Answer from the drawing. Dimensions are ordinates in mm from the lowest x, y and z of the part. A direction names the side the tool comes from. Coordinates: 2 decimals unless noted, no trailing zeros. Write each loop counter-clockwise with the first axis right and the second up, starting at its lowest first coordinate (ties: lowest second). Pieces come first, ordered by that corner, then holes.
1) The part is cut by section B-B (y = 10). Determine the outline of the cut face in (x, z).
2) Find the intervals of material crossed by line 1 (X direction, y = 9.25, z = 13); line 2 (Y direction, x = 12.7, z = 11.5); line 3 (Y direction, x = 15.5, z = 9.5), in increasing order.
3) Which of the six approach directions +Z, -Z, +X, -X, +Y, -Y give full straight-line access (tool end or side, diameter ignored) to the marked faces 1, 2 and 3?
4) The part is cut by section C-C (x = 21.5). Determine the outline of the cut face in (y, z).
5) Each of these flat-tipped pins is pushed along its axis until it touches: pin 1 Ø6 at (x, z) = (10, 5.5) entering from +Y; pin 2 Ø1.9 at (y, z) = (6, 7.5) entering from +X; pin 3 Ø3 at (y, z) = (6, 5) entering from -X; pin 4 Ø5.5 at (x, z) = (3.048, 7.62) entering from +Y. Where does it stop, or does it pass through?
6) The part is cut by section A-A (z = 9.5). Give the number of separate pieces and of enclosed holes in the cut face, then the cut area to 3 significant figures.
7) Determine the mould class of the marked faces 4, 5 and 6 for opening direction X: +X half, -X half, draft (parallel to the pull), parting line (faces both ways), or undercut.
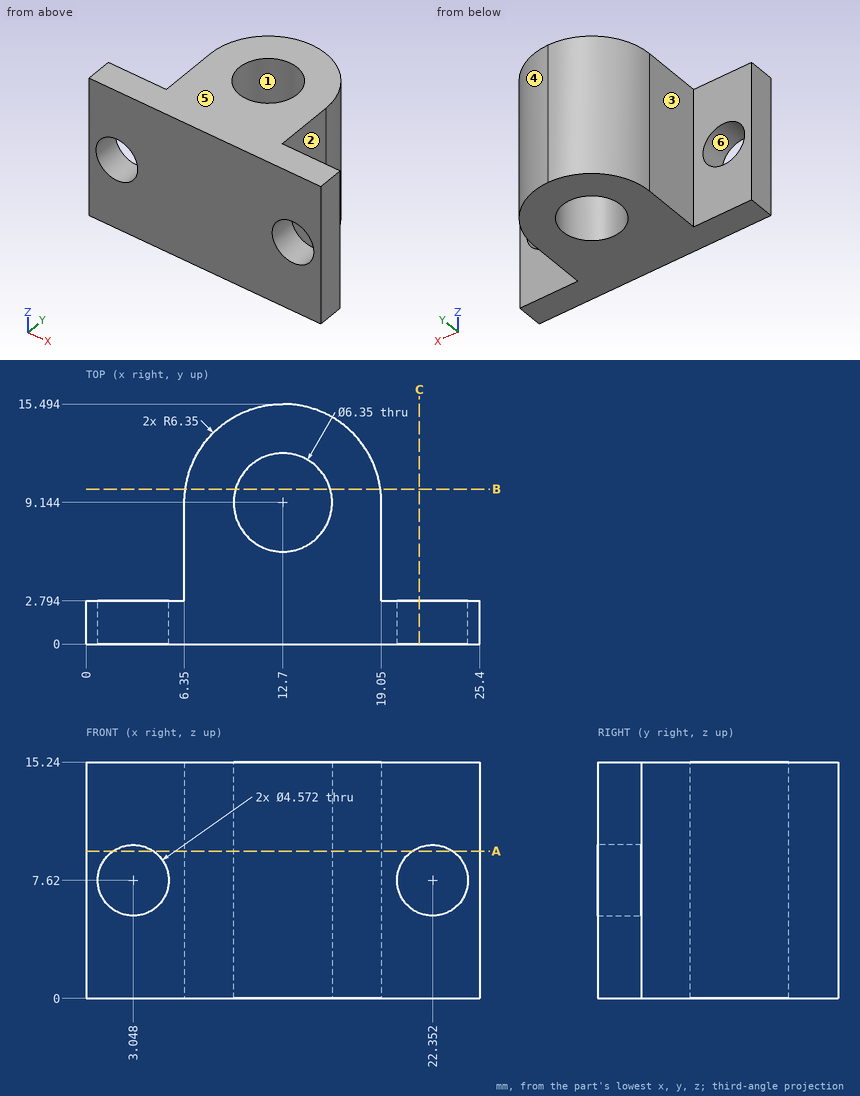
Reported:
1. outline: (6.41, 0) - (9.64, 0) - (9.64, 15.24) - (6.41, 15.24) - close; (15.76, 0) - (18.99, 0) - (18.99, 15.24) - (15.76, 15.24) - close
2. line 1: x = 6.35 to 9.53, 15.87 to 19.05
2. line 2: y = 0 to 5.97, 12.32 to 15.49
2. line 3: y = 0 to 7.65, 10.64 to 14.84
3. face 1: +Z, -Z
3. face 2: +Z, -Z, +X, +Y
3. face 3: +Z, -Z, -X, +Y
4. outline: (0, 0) - (2.79, 0) - (2.79, 5.5) - (0, 5.5) - close; (0, 9.74) - (2.79, 9.74) - (2.79, 15.24) - (0, 15.24) - close
5. pin 1: stops at y = 15.49
5. pin 2: stops at x = 19.05
5. pin 3: stops at x = 6.35
5. pin 4: stops at y = 2.79
6. separate pieces: 3
6. enclosed holes: 1
6. area: 169 mm2
7. face 4: +X half
7. face 5: draft
7. face 6: undercut
